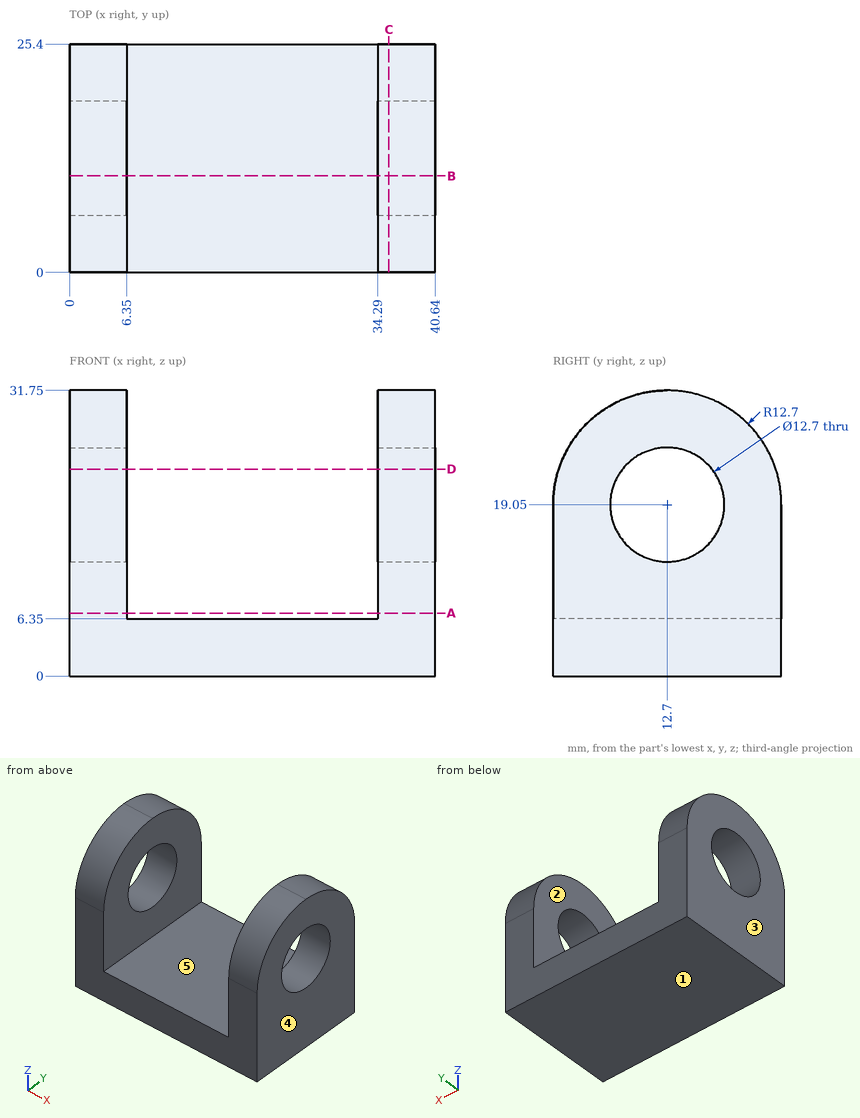
The drawing under review shows one solid part. Ordinate dimensions are in mm from its lowest x, y, z. A direction names the side the tool comes from. Round coordinates to 2 decimals unless told otherwise and drop trailing zeros. Write each loop counter-clockwise with the first axis right and the second up, starting at its lowest first coordinate (ties: lowest second). Pieces come first, ordered by that corner, then holes. Notation, with made-up numbers: M 63.25,45 L 103.25,45 A15 cw 103.25,57 Z; hole C 69.25,38 d10. An arc over 180 degrees is marked long. One line per item, written item: value. Start each with the question number.
(1) The part is to be moulded in two halves that separate along X. For the marked faces 3, 4 and 5, say which applies: released by +X, released by -X, zero draft, split by the parting line, or undercut.
(2) We need section C-C (x = 35.5). Give the boundary of the cut face in (y, z).
(3) We need section A-A (z = 7). Give the boundary of the cut face in (x, y).
(4) We need section B-B (y = 10.75). Give the boundary of the cut face in (x, z).
(5) Wall thickness on line 1 (X direction, y = 20.25, z = 7); line 2 (Z direction, x = 2, y = 12.7); line 3 (Z direction, x = 13, y = 15.5): over which ranges is each line inside the solid? List them lowest first.
(6) Machinability: for the marked faces 1 and 2, which of the approach directions +Z, -Z, +X, -X, +Y, -Y give a long, thin tool a straight path to every point of the face, cutting with its end or side? Answer none if there is none.
(7) We need section D-D (z = 23). Give the boundary of the cut face in (x, y), and give its area (3 significant figures).
(8) Insertion check: pin 1 (1.5 mm diameter, centred on x = 30.5, y = 16.5, fed in from +Z); pin 2 (4 mm diameter, centred on x = 4.5, y = 17, fed in from +Z). Each pin has a flat end and moves straight along its axis. Give the tip position at first contact, or say it passes through.
Result:
1. face 3: released by -X
1. face 4: released by +X
1. face 5: undercut
2. outline: M 0,0 L 25.4,0 L 25.4,19.05 A12.7 ccw 0,19.05 Z; hole C 12.7,19.05 d12.7
3. outline: M 0,0 L 6.35,0 L 6.35,25.4 L 0,25.4 Z; M 34.29,0 L 40.64,0 L 40.64,25.4 L 34.29,25.4 Z
4. outline: M 0,0 L 40.64,0 L 40.64,13.01 L 34.29,13.01 L 34.29,6.35 L 6.35,6.35 L 6.35,13.01 L 0,13.01 Z; M 0,25.09 L 6.35,25.09 L 6.35,31.6 L 0,31.6 Z; M 34.29,25.09 L 40.64,25.09 L 40.64,31.6 L 34.29,31.6 Z
5. line 1: 0 to 6.35, 34.29 to 40.64
5. line 2: 0 to 12.7, 25.4 to 31.75
5. line 3: 0 to 6.35
6. face 1: -Z, +X, -X, +Y, -Y
6. face 2: +Z, +Y, -Y
7. outline: M 0,0.63 L 6.35,0.63 L 6.35,7.73 L 0,7.73 Z; M 0,17.67 L 6.35,17.67 L 6.35,24.77 L 0,24.77 Z; M 34.29,0.63 L 40.64,0.63 L 40.64,7.73 L 34.29,7.73 Z; M 34.29,17.67 L 40.64,17.67 L 40.64,24.77 L 34.29,24.77 Z
7. area: 180 mm²
8. pin 1: z = 6.35
8. pin 2: z = 31.54
